Part model, mm, in its own coordinate system. Face numbers are marked on the shaded views. Give positions to 0.01 mm unless a question says otherwise; leave off trailing zeros. Write each loop counter-clockwise with the first axis right and the second up, starting at its lowest first coordinate (ties: lowest second). Pieces come first, ordered by that corner, then holes. Notation, with made-up numbers: (-24, -35.5) - (-3, -35.5) arc R25 cw to (-3, -11.5) - close; hole circle Ø9 at (81, 14.5). An arc over 180 degrees is marked (long way). Answer as a JSON object with one key per item and string values. Group by question number.
```python
from build123d import *

# Parameters (mm, degrees)
F1_W     = 151.38457
F1_H     = 151.737027
F2_DEPTH = 246.634
F3_R     = 20.32
F4_W     = 123.892136
F4_H     = 124.420833
F5_DEPTH = 238.252
F6_W     = 151.38457
F6_H     = 246.634
F7_DEPTH = 0.762
F8_R     = 7.823659
F9_DEPTH = 130.302


with BuildPart() as f2:
    # F1 (on offset) → F2 (new body)
    with BuildSketch(Plane.XY.offset(-76.454)):
        with Locations((4e-06, -0.176233)):
            Rectangle(F1_W, F1_H)
    extrude(amount=F2_DEPTH)

    # F3
    f3_edges = [f2.edges().sort_by_distance(p)[0] for p in [
        (4e-06, 75.692281, 170.18),
        (75.692289, 75.692281, 46.863),
        (4e-06, 75.692281, -76.454),
        (-75.692281, 75.692281, 46.863),
    ]]
    fillet(f3_edges, radius=F3_R)

    # F4 (on face) → F5 (cut)
    with BuildSketch(Plane.XY.offset(170.18)):
        with Locations((1.057398, -13.83433)):
            Rectangle(F4_W, F4_H)
    extrude(amount=-F5_DEPTH, mode=Mode.SUBTRACT)

    # F6 (on face) → F7 (join)
    with BuildSketch(Plane.XZ.offset(76.044746)):
        with Locations((4e-06, 46.863)):
            Rectangle(F6_W, F6_H)
    extrude(amount=F7_DEPTH)

    # F8 (on face) → F9 (join)
    with BuildSketch(Plane.YZ.offset(-60.88867)):
        with Locations((-18.548923, -6.748606)):
            Circle(F8_R)
    extrude(amount=F9_DEPTH)


solid = f2.part
```
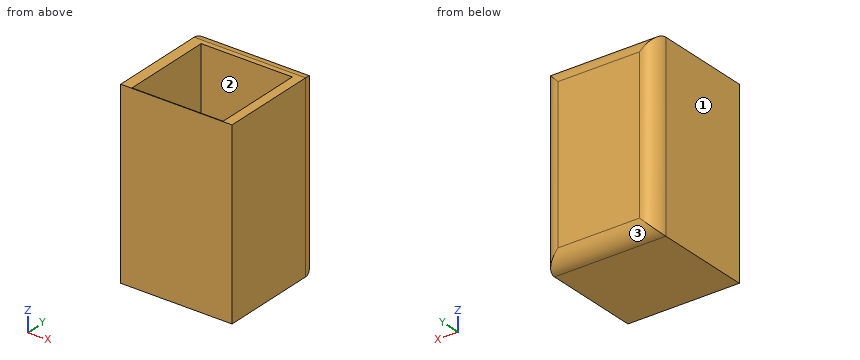
1) Drop a flat-ended pin along its axis: P1, Ø10, axis at x = 23.5, y = 10, coming from the +Z side. Give the stop position or say it passes through.
2) Saw through at D-D (y = 42.5). List the corners of the cut face in (x, z).
3) Saw through at A-A (z = 49). List the corners of the cut face in (x, y), and give its area (3 significant figures).
4) Drill centre lines: line 1 along Y through (x, z) = (29.5, 20); line 2 along X through (y, z) = (27.5, 147); line 3 along Z through (x, y) = (-46, -64). Where is each one in solid material? Low to high. Write a range as from..to.
5) Saw through at B-B (y = -14.5). List the corners of the cut face in (x, z), and give its area (3 significant figures).
6) Two-plate mould, pull along Y, no slides. Class the marked faces 1, 2 and 3: +Y half, -Y half, draft (parallel to the pull), parting line (faces both ways), or undercut.
7) Saw through at C-C (x = 32.5). List the corners of the cut face in (y, z).
Checks:
{
 "1": {"P1": "z = -68.07"},
 "2": {"outline": "(-75.69, -76.45) - (75.69, -76.45) - (75.69, 170.18) - (63, 170.18) - (63, -68.07) - (-60.89, -68.07) - (-60.89, 170.18) - (-75.69, 170.18) - close"},
 "3": {"outline": "(-75.69, -76.81) - (75.69, -76.81) - (75.69, 55.37) arc R20.32 ccw to (55.37, 75.69) - (-55.37, 75.69) arc R20.32 ccw to (-75.69, 55.37) - close; hole (-60.89, -76.04) - (63, -76.04) - (63, 48.38) - (-60.89, 48.38) - close", "area": "7,490 mm2"},
 "4": {"line 1": "-76.81..-76.04, 48.38..75.69", "line 2": "-75.69..-60.89, 63..75.69", "line 3": "-76.45..-68.07"},
 "5": {"outline": "(-75.69, -76.45) - (75.69, -76.45) - (75.69, 170.18) - (63, 170.18) - (63, -0.05) - (-60.89, -0.05) - (-60.89, 170.18) - (-75.69, 170.18) - close; hole (-60.89, -68.07) - (63, -68.07) - (63, -13.44) - (-60.89, -13.44) - close", "area": "9,480 mm2"},
 "6": {"face 1": "draft", "face 2": "undercut", "face 3": "+Y half"},
 "7": {"outline": "(-76.81, -76.45) - (55.37, -76.45) arc R20.32 ccw to (75.69, -56.13) - (75.69, 149.86) arc R20.32 ccw to (55.37, 170.18) - (48.38, 170.18) - (48.38, -68.07) - (-76.04, -68.07) - (-76.04, 170.18) - (-76.81, 170.18) - close; circle Ø15.65 at (-18.55, -6.75)"}
}
